Can you work these out from the model? Positions are in its coordinate system, mm. A direction names the side the tool comes from. Coordinates: 2 decimals unless noted, no trailing zeros. Order: outer loops, then holes, each group sorted by start corner. A loop starts at its lowest first (then second) coordinate and runs counter-clockwise, first axis right, second up.
Autodesk Inventor part; units mm, degrees
ref_plane "YZ Plane" through (0, 0, 0) normal (1, 0, 0) x (0, 1, 0)
ref_plane "XZ Plane" through (0, 0, 0) normal (0, 1, 0) x (-1, 0, 0)
ref_plane "XY Plane" through (0, 0, 0) normal (0, 0, 1) x (1, 0, 0)
sketch "스케치1" plane through (0, 0, 0) normal (0, 0, 1) x (1, 0, 0)
  line L0 (-9.25, 0) -> (9.25, 0)
  arc A0 (9.25, 0) -> (-9.25, 0) centre (0, 0) ccw
  line L1 (0, 9.25) -> (0, 0) construction
  line L2 (-6, 0) -> (6, 0)
  line L3 (6, 0) -> (6, -13)
  line L4 (6, -13) -> (-6, -13)
  line L5 (-6, -13) -> (-6, 0)
  dimension "d0" = 18.5
  dimension "d1" = 9.25
  dimension "d2" = 12
  dimension "d3" = 13
extrude "돌출1" add sketch "스케치1" along normal mid plane 7 contours A0 L0
extrude "돌출2" add sketch "스케치1" along normal mid plane 4.5 contours L0 L3 L4 L5
properties part number "Mic"
1. On a 3-axis mill with a long thin cutter (end or side, diameter ignored), from which of +Z, -Z, +X, -X, +Y, -Y can I reach the whole of each face in a straight line? I mean faces 1 (the flat face through (0, -6, 2.25)), 2 (the flat face through (6, -6, 0)), 3 (the flat face through (-6, -7, 0)). Say none if no direction works.
Completed:
face 1: +Z, +X, -X, -Y
face 2: +Z, -Z, +X, -Y
face 3: +Z, -Z, -X, -Y
2. Please list where these lines run through material, in increasing order: probe 1 along X at (y, z) = (-3.25, 0); probe 2 along Z at (x, y) = (4, -9.5); probe 3 along Y at (x, z) = (7.5, -1.75).
Completed:
probe 1: x = -6 to 6
probe 2: z = -2.25 to 2.25
probe 3: y = 0 to 5.41
3. Imagine slicing it at B-B on z = -1. Please give me the cut outline in (x, y).
Completed:
outline: (-9.25, 0) - (-6, 0) - (-6, -13) - (6, -13) - (6, 0) - (9.25, 0) arc R9.25 ccw to start
4. Imagine slicing it at D-D on x = -5.5. Please give me the cut outline in (y, z), then the cut area to 3 significant figures.
Completed:
outline: (-13, -2.25) - (0, -2.25) - (0, -3.5) - (7.44, -3.5) - (7.44, 3.5) - (0, 3.5) - (0, 2.25) - (-13, 2.25) - close
area: 111 mm2
5. Imagine slicing it at C-C on y = 3. Please give me the cut outline in (x, z).
Completed:
outline: (-8.75, -3.5) - (8.75, -3.5) - (8.75, 3.5) - (-8.75, 3.5) - close
6. Imagine slicing it at A-A on x = 0. Please give me the cut outline in (y, z).
Completed:
outline: (-13, -2.25) - (0, -2.25) - (0, -3.5) - (9.25, -3.5) - (9.25, 3.5) - (0, 3.5) - (0, 2.25) - (-13, 2.25) - close
7. I'm going to push flat-ended pins straight in: pin 1 (4 mm diameter, centred on y = 5.5, z = 0, fed in from -X); pin 2 (9.5 mm diameter, centred on x = -1.5, y = -6.5, fed in from -Z); pin 3 (3.5 mm diameter, centred on y = -8, z = 0, fed in from +X). Where does each tip first touch, or does it pass through?
Completed:
pin 1: stops at x = -8.56
pin 2: stops at z = -2.25
pin 3: stops at x = 6
